Verification items for this drawing (mm, ordinates from the low corner). A direction names the side the tool comes from. Coordinates: 2 decimals unless noted, no trailing zeros. Order: outer loops, then holes, each group sorted by start corner. A loop starts at its lowest first (then second) coordinate and runs counter-clockwise, first axis right, second up. Notation, with made-up numbers: (23, -37) -> (72, -37) arc R27 ccw to (72, -4) -> close; hole circle Ø1 at (66.5, -25). An arc over 180 degrees is marked (long way). Answer in a Markdown table with one row per item. Add a question column.
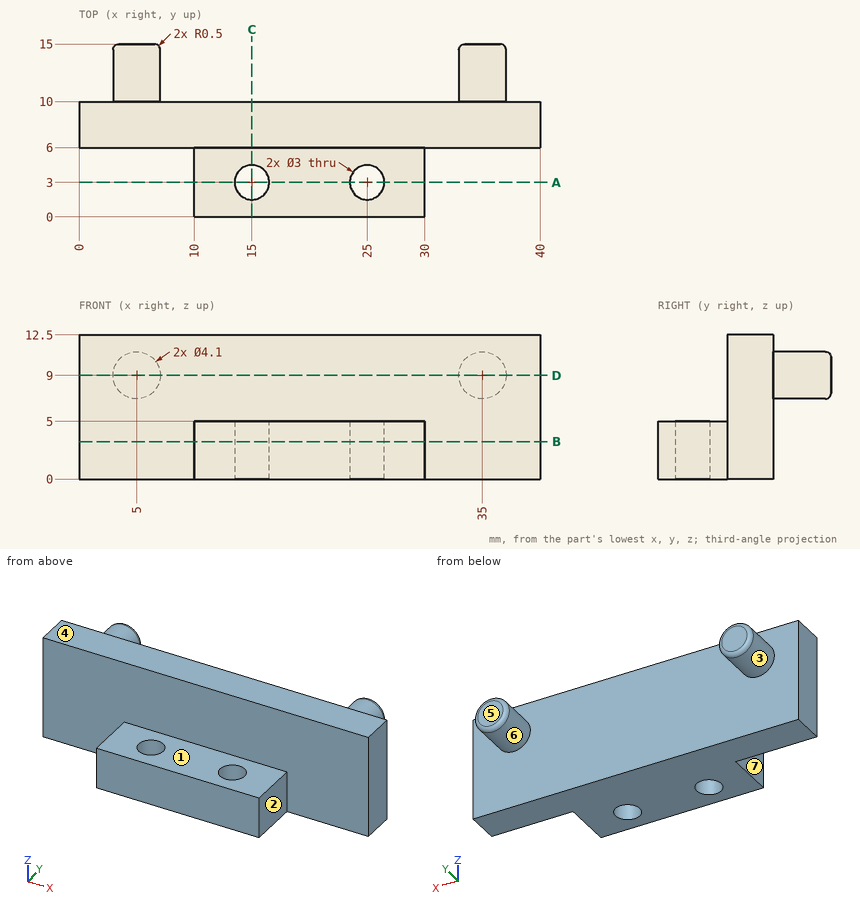
(1) Go/stop test with flat-tipped pins: P1, Ø1.5, axis at y = 3.5, z = 3.5, coming from the -X side; P2, Ø1.8, axis at x = 19.5, y = 4, coming from the +Z side; P3, Ø1.5, axis at y = 3, z = 2, coming from the +X side. Record where each tip stops, or that it passes through.
(2) Cross-section at D-D (z = 9). Enter the section's corners in (x, y).
(3) Cross-section at A-A (y = 3). Enter the section's corners in (x, z), plus the area to 3 significant figures.
(4) Mould release check, pull along X, two halves, no side actions. Record for the marked faces 5, 6 and 7: +X half, -X half, draft (parallel to the pull), parting line (faces both ways), or undercut.
(5) Scan lines: line 1 along Y through (x, z) = (15, 2.25); line 2 along X through (y, z) = (1.75, 4.5); line 3 along Y through (x, z) = (20, 5.5). Record each from-to range of solid material in increasing order.
(6) Cross-section at B-B (z = 3.25). Enter the section's corners in (x, y), plus the area to 3 significant figures.
(7) Access from +Z, -Z, +X, -X, +Y, -Y to the whole of each face (thin tool, end or side, straight path). Record for the marked faces 1, 2, 3 and 4.
(8) Cross-section at C-C (x = 15). Enter the section's corners in (y, z).
Checks:
| question | item | result |
|---|---|---|
| 1 | P1 | x = 10 |
| 1 | P2 | z = 5 |
| 1 | P3 | x = 30 |
| 2 | outline | (0, 6) -> (40, 6) -> (40, 10) -> (37.05, 10) -> (37.05, 14.5) arc R0.5 ccw to (36.55, 15) -> (33.45, 15) arc R0.5 ccw to (32.95, 14.5) -> (32.95, 10) -> (7.05, 10) -> (7.05, 14.5) arc R0.5 ccw to (6.55, 15) -> (3.45, 15) arc R0.5 ccw to (2.95, 14.5) -> (2.95, 10) -> (0, 10) -> close |
| 3 | outline | (10, 0) -> (13.5, 0) -> (13.5, 5) -> (10, 5) -> close; (16.5, 0) -> (23.5, 0) -> (23.5, 5) -> (16.5, 5) -> close; (26.5, 0) -> (30, 0) -> (30, 5) -> (26.5, 5) -> close |
| 3 | area | 70.0 mm² |
| 4 | face 5 | draft |
| 4 | face 6 | undercut |
| 4 | face 7 | -X half |
| 5 | line 1 | 0 to 1.5, 4.5 to 10 |
| 5 | line 2 | 10 to 14.17, 15.83 to 24.17, 25.83 to 30 |
| 5 | line 3 | 6 to 10 |
| 6 | outline | (0, 6) -> (10, 6) -> (10, 0) -> (30, 0) -> (30, 6) -> (40, 6) -> (40, 10) -> (0, 10) -> close; hole circle Ø3 at (15, 3); hole circle Ø3 at (25, 3) |
| 6 | area | 266 mm² |
| 7 | face 1 | +Z, +X, -X, -Y |
| 7 | face 2 | +Z, -Z, +X, -Y |
| 7 | face 3 | +Y |
| 7 | face 4 | +Z, +X, -X, +Y, -Y |
| 8 | outline | (0, 0) -> (1.5, 0) -> (1.5, 5) -> (0, 5) -> close; (4.5, 0) -> (10, 0) -> (10, 12.5) -> (6, 12.5) -> (6, 5) -> (4.5, 5) -> close |
